The model under review builds one solid part; all positions refer to its coordinate system, in mm. A direction names the side the tool comes from. Coordinates: 2 decimals unless noted, no trailing zeros. Order: outer loops, then holes, each group sorted by start corner. A loop starts at its lowest first (then second) coordinate and runs counter-clockwise, first axis right, second up. Notation, with made-up numbers: (-3, 83.25) -> (19, 83.25) arc R12 cw to (19, 105.25) -> close; hole circle Ø8 at (13.25, 49.25). An arc over 180 degrees is marked (long way). Put each result on its own line as item: value.
from build123d import *

# Parameters (mm, degrees)
SKETCH_1_W          = 92
SKETCH_1_H          = 60
SKETCH_1_R          = 2.5
SKETCH_1_R_2        = 5
SKETCH_1_R_3        = 3
EXTRUDE_1_DEPTH     = 4
SKETCH_2_W          = 10
SKETCH_2_H          = 15
CUT_EXTRUDE_1_DEPTH = 10
CUT_EXTRUDE_2_DEPTH = 4


with BuildPart() as part:
    # Эскиз1 → Бобышка-Вытянуть1 (new body)
    with BuildSketch(Plane(origin=(0, 0, 0), x_dir=(1, 0, 0), z_dir=(0, 1, 0))):
        with Locations((46, 30)):
            Rectangle(SKETCH_1_W, SKETCH_1_H)
        with Locations(Location((12, 50, 0), (0, 0, 270))):
            Circle(SKETCH_1_R, mode=Mode.SUBTRACT)
        with Locations(Location((12, 20, 0), (0, 0, 270))):
            Circle(SKETCH_1_R, mode=Mode.SUBTRACT)
        with Locations(Location((80, 50, 0), (0, 0, 270))):
            Circle(SKETCH_1_R, mode=Mode.SUBTRACT)
        with Locations(Location((80, 20, 0), (0, 0, 270))):
            Circle(SKETCH_1_R, mode=Mode.SUBTRACT)
        with Locations(Location((29, 25, 0), (0, 0, 270))):
            Circle(SKETCH_1_R_2, mode=Mode.SUBTRACT)
        with Locations(Location((63, 25, 0), (0, 0, 270))):
            Circle(SKETCH_1_R_2, mode=Mode.SUBTRACT)
        with Locations(Location((29, 41, 0), (0, 0, 270))):
            Circle(SKETCH_1_R_3, mode=Mode.SUBTRACT)
        with Locations(Location((29, 9, 0), (0, 0, 270))):
            Circle(SKETCH_1_R_3, mode=Mode.SUBTRACT)
        with Locations(Location((63, 41, 0), (0, 0, 270))):
            Circle(SKETCH_1_R_3, mode=Mode.SUBTRACT)
        with Locations(Location((63, 9, 0), (0, 0, 270))):
            Circle(SKETCH_1_R_3, mode=Mode.SUBTRACT)
    extrude(amount=EXTRUDE_1_DEPTH)

    # Эскиз2 → Вырез-Вытянуть1 (cut)
    with BuildSketch(Plane(origin=(0, 4, 0), x_dir=(1, 0, 0), z_dir=(0, 1, 0))):
        with Locations((46, 7.5)):
            Rectangle(SKETCH_2_W, SKETCH_2_H)
    extrude(amount=-CUT_EXTRUDE_1_DEPTH, mode=Mode.SUBTRACT)

    # Эскиз3 → Вырез-Вытянуть2 (cut)
    with BuildSketch(Plane(origin=(0, 4, 0), x_dir=(1, 0, 0), z_dir=(0, 1, 0))):
        Polygon((10, 0), (0, 10), (0, 0), align=None)
        Polygon((92, 0), (92, 10), (82, 0), align=None)
    extrude(amount=-CUT_EXTRUDE_2_DEPTH, mode=Mode.SUBTRACT)


solid = part.part
Item 1: Consider section A-A on z = -9. Write out the cut boundary in (x, y), and give its area (3 significant figures).
Answers below:
outline: (1, 0) -> (26, 0) -> (26, 4) -> (1, 4) -> close; (32, 0) -> (41, 0) -> (41, 4) -> (32, 4) -> close; (51, 0) -> (60, 0) -> (60, 4) -> (51, 4) -> close; (66, 0) -> (91, 0) -> (91, 4) -> (66, 4) -> close
area: 272 mm^2
Item 2: Consider section B-B on x = 63. Write out the cut boundary in (y, z).
Answers below:
outline: (0, -60) -> (4, -60) -> (4, -44) -> (0, -44) -> close; (0, -38) -> (4, -38) -> (4, -30) -> (0, -30) -> close; (0, -20) -> (4, -20) -> (4, -12) -> (0, -12) -> close; (0, -6) -> (4, -6) -> (4, 0) -> (0, 0) -> close
Item 3: Consider section C-C on z = -48.5. Write out the cut boundary in (x, y).
Answers below:
outline: (0, 0) -> (10, 0) -> (10, 4) -> (0, 4) -> close; (14, 0) -> (78, 0) -> (78, 4) -> (14, 4) -> close; (82, 0) -> (92, 0) -> (92, 4) -> (82, 4) -> close
Item 4: Mouldability with a two-part tool opening along Z and no side actions: class faces 1 (the cylindrical face through (9.78, 1.97, -48.85)), 2 (the flat face through (45, 2, -60)), 3 (the flat face through (5, 2, -5)), 4 (the flat face through (51, 2, -7)) as +Z half, -Z half, draft (parallel to the pull), parting line (faces both ways), or undercut.
Answers below:
face 1: undercut
face 2: -Z half
face 3: +Z half
face 4: draft
Item 5: For pin 1 Ø2 at (x, y) = (47.5, 3) entering from +Z, flat-tipped, find the tip position at first contact; note if it passes through.
Answers below:
pin 1: z = -15
Item 6: For faces 5 (the flat face through (46, 2, -15)), 6 (the flat face through (45, 0, -30)), list the 3-axis set-ups (+Z, -Z, +X, -X, +Y, -Y) from which the entire face can be reached by the end or side of a thin tool; tool diameter is ignored.
Answers below:
face 5: +Z, +Y, -Y
face 6: +Z, -Z, +X, -X, -Y
Item 7: Consider section D-D on y = 2.1. Count the separate pieces of the cut face and the enclosed holes in it, and give its area (3 significant figures).
Answers below:
separate pieces: 1
enclosed holes: 10
area: 4,920 mm^2
Item 8: For line 1 (X direction, y = 2.8, z = -25); line 2 (X direction, y = 1.25, z = -50); line 3 (X direction, y = 0.4, z = -8.5), list the stretches that pass through material, from the lowest coordinate up. Write a range as from..to.
Answers below:
line 1: 0..24, 34..58, 68..92
line 2: 0..9.5, 14.5..77.5, 82.5..92
line 3: 1.5..26.04, 31.96..41, 51..60.04, 65.96..90.5
